Read the model definition and answer for the solid it produces. Units are mm, in the model's axes. Round coordinates to 2 decimals unless told otherwise and drop trailing zeros. Loops run counter-clockwise (first coordinate to the right, second up) from the corner with the lowest first, then second, coordinate; pieces in that order, holes last. Notation, with made-up numbers: (-30.75, 32) - (16.25, 32) arc R21 ccw to (16.25, 60) - close; hole circle Ø3 at (50, 83.25). An arc over 180 degrees is marked (long way). Use CSV: the item, a comma, the result in double quotes. Start each with the question number.
1. Consider line 1 along Z through (x, y) = (-12, 0); line 2 along X through (y, z) = (-2.5, 3.15) (3 decimals); line 3 along X through (y, z) = (-2, 2.55). Determine where each line is inside the solid, lowest interval first.
2. Find section D-D (x = 7). Give the vertices of the cut face in (y, z).
3. Find section B-B (z = 1.2). Give the vertices of the cut face in (x, y) (3 decimals), and give its area (3 significant figures).
4. Determine the mould class of faces 1 (the cylindrical face through (-3, 0, 2)), 2 (the flat face through (9, 0, 1.5)), 3 (the flat face through (-8.28, 2.38, 0.74)) for opening direction X: +X half, -X half, draft (parallel to the pull), parting line (faces both ways), or undercut.
5. Given pin 1 Ø1.5 at (x, z) = (-11, 2.5) entering from -Y; pin 2 Ø1 at (x, y) = (10.5, 1.5) entering from +Z, each flat-ended and moving along its own axis, determine where each tip first touches the part or whether it passes through.
6. Find section A-A (x = 0). Give the vertices of the cut face in (y, z) (3 decimals), and give its area (4 significant figures).
7. Find section C-C (y = -1.25). Give the vertices of the cut face in (x, z).
from build123d import *

# Parameters (mm, degrees)
F0_R     = 3
F1_DEPTH = 3.5
F2_DEPTH = 1.5


with BuildPart() as f1:
    # F0 (on Top) → F1 (new body)
    with BuildSketch(Plane.XY):
        with BuildLine():
            ThreePointArc((2.361805, -2.75), (3.294098, -1.513123), (3.625, 0))
            ThreePointArc((3.625, 0), (3.294098, 1.513123), (2.361805, 2.75))
            ThreePointArc((2.361805, 2.75), (0, 3.625), (-2.361805, 2.75))
            ThreePointArc((-2.361805, 2.75), (-3.625, 0), (-2.361805, -2.75))
            ThreePointArc((-2.361805, -2.75), (0, -3.625), (2.361805, -2.75))
        make_face()
        Circle(F0_R, mode=Mode.SUBTRACT)
    extrude(amount=F1_DEPTH)

    # F0 (on Top) → F2 (join)
    with BuildSketch(Plane.XY):
        with BuildLine():
            ThreePointArc((-2.361805, -2.75), (-3.625, 0), (-2.361805, 2.75))
            Line((-2.361805, 2.75), (-14.375267, 1.996073))
            ThreePointArc((-14.375267, 1.996073), (-12.880791, 1.45783), (-12.25, 0))
            ThreePointArc((-12.25, 0), (-12.880791, -1.45783), (-14.375267, -1.996073))
            Line((-14.375267, -1.996073), (-2.361805, -2.75))
        make_face()
        with BuildLine():
            ThreePointArc((-12.25, 0), (-12.880791, 1.45783), (-14.375267, 1.996073))
            ThreePointArc((-14.375267, 1.996073), (-16.25, 0), (-14.375267, -1.996073))
            ThreePointArc((-14.375267, -1.996073), (-12.880791, -1.45783), (-12.25, 0))
        make_face()
        with BuildLine():
            ThreePointArc((2.361805, 2.75), (3.294098, 1.513123), (3.625, 0))
            ThreePointArc((3.625, 0), (3.294098, -1.513123), (2.361805, -2.75))
            Line((2.361805, -2.75), (14.375267, -1.996073))
            ThreePointArc((14.375267, -1.996073), (12.25, 0), (14.375267, 1.996073))
            Line((14.375267, 1.996073), (2.361805, 2.75))
        make_face()
        with BuildLine():
            ThreePointArc((16.25, 0), (15.70783, 1.369209), (14.375267, 1.996073))
            ThreePointArc((14.375267, 1.996073), (12.25, 0), (14.375267, -1.996073))
            ThreePointArc((14.375267, -1.996073), (15.70783, -1.369209), (16.25, 0))
        make_face()
    extrude(amount=F2_DEPTH)


solid = f1.part
Filled sheet:
1,line 1,"z = 0 to 1.5"
1,line 2,"x = -2.625 to -1.658, 1.658 to 2.625"
1,line 3,"x = -3.02 to -2.24, 2.24 to 3.02"
2,outline,"(-2.46, 0) - (2.46, 0) - (2.46, 1.5) - (-2.46, 1.5) - close"
3,outline,"(-14.375, -1.996) - (-2.362, -2.75) arc R3.625 ccw to (2.362, -2.75) - (14.375, -1.996) arc R2 ccw to (16.25, 0) arc R2 ccw to (14.375, 1.996) - (2.362, 2.75) arc R3.625 ccw to (-2.362, 2.75) - (-14.375, 1.996) arc R2 ccw to start; hole circle Ø6 at (0, 0)"
3,area,"129 mm²"
4,face 1,"undercut"
4,face 2,"draft"
4,face 3,"-X half"
5,pin 1,"passes through"
5,pin 2,"stops at z = 1.5"
6,outline,"(-3.625, 0) - (-3, 0) - (-3, 3.5) - (-3.625, 3.5) - close; (3, 0) - (3.625, 0) - (3.625, 3.5) - (3, 3.5) - close"
6,area,"4.375 mm²"
7,outline,"(-15.81, 0) - (-2.73, 0) - (-2.73, 3.5) - (-3.4, 3.5) - (-3.4, 1.5) - (-15.81, 1.5) - close; (2.73, 0) - (15.81, 0) - (15.81, 1.5) - (3.4, 1.5) - (3.4, 3.5) - (2.73, 3.5) - close"
